Can you work these out from the model? Positions are in its coordinate system, mm. Face numbers are marked on the shaded views. A direction names the side the tool comes from. Coordinates: 2 decimals unless noted, no trailing zeros. Order: outer loops, then holes, each group sorted by start corner. A loop starts at its lowest first (then second) coordinate and runs counter-clockwise, first axis right, second up. Notation, with made-up numbers: (31, 0.25) -> (55, 0.25) arc R22 cw to (55, 18.25) -> close; hole circle Ø6 at (25, -16.5). An arc over 180 degrees is marked (long way). Answer in a Markdown table with one row per item. Add a question column.
1. We'd pull the mould along Z, two halves only. Please class the marked faces 1, 2, 3 and 4: pulls with the +Z half, pulls with the -Z half, needs draft (parallel to the pull), parting line crosses it, or undercut.
2. Imagine slicing it at C-C on z = 36. Write out the boundary of the cut face in (x, y).
3. Imagine slicing it at B-B on y = 45. Write out the boundary of the cut face in (x, z).
4. Imagine slicing it at A-A on x = 16. State how many separate pieces and enclosed holes the cut face has, plus the area to 4 significant figures.
5. Will these pins go through, and if not, where does the flat tip stop? pin 1 (10 mm diameter, centred on y = 33, z = 23.5, fed in from -X); pin 2 (3 mm diameter, centred on x = 22.5, z = 13.5, fed in from +Y); pin 3 (5 mm diameter, centred on x = 36, z = 16, fed in from -Y); pin 4 (2.5 mm diameter, centred on x = 16, y = 47.5, fed in from +Z).
6. Imagine slicing it at D-D on y = 27. Write out the boundary of the cut face in (x, z).
7. On a 3-axis mill with a long thin cutter (end or side, diameter ignored), from which of +Z, -Z, +X, -X, +Y, -Y can I reach the whole of each face in a straight line? I mean the marked faces 5 and 6. Say none if no direction works.
8. If I drill on line 1 along Z through (x, y) = (6.55, 16); line 2 along Z through (x, y) = (6.5, 29.5), over which ranges is the centre line in solid material (lowest first)? Write a range as [from, to].
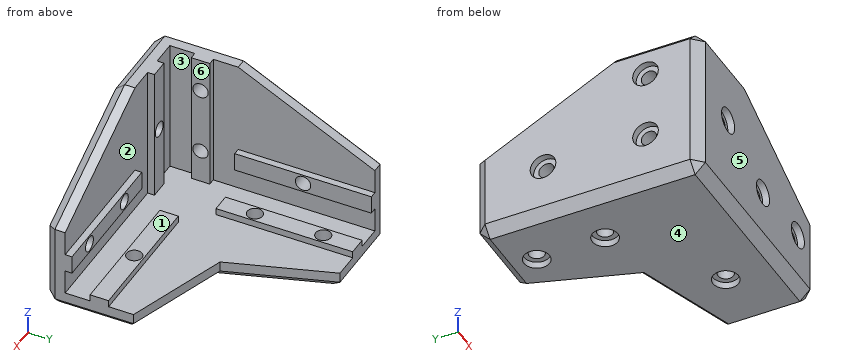
from build123d import *

# Parameters (mm, degrees)
F1_DEPTH  = 6
F3_DEPTH  = 20
F5_DEPTH  = 20
F7_DEPTH  = 40
F9_DEPTH  = 2
F11_DEPTH = 2
F13_DEPTH = 2
F14_R     = 2.25
F15_DEPTH = 8
F16_R     = 2.25
F17_DEPTH = 8
F18_R     = 2.25
F19_DEPTH = 8
F20_R     = 3.75
F21_DEPTH = 2
F22_R     = 3.75
F23_DEPTH = 2
F24_R     = 3.75
F25_DEPTH = 2
F27_DEPTH = 6
F29_DEPTH = 6
F31_DEPTH = 6
F32_SIZE  = 3


with BuildPart() as f1:
    # F0 (on Top) → F1 (new body)
    with BuildSketch(Plane.XY):
        Polygon((0, 66), (0, 0), (66, 0), (66, 26), (26, 26), (26, 66), align=None)
    extrude(amount=F1_DEPTH)

    # F2 (on face) → F3 (join)
    with BuildSketch(Plane.XY.offset(6)):
        Polygon((6, 66), (0, 66), (0, 0), (66, 0), (66, 6), (6, 6), align=None)
    extrude(amount=F3_DEPTH)

    # F4 (on face) → F5 (join)
    with BuildSketch(Plane.XY.offset(26)):
        Polygon((6, 6), (6, 26), (0, 26), (0, 0), (26, 0), (26, 6), align=None)
    extrude(amount=F5_DEPTH)

    # F6 (on face) → F7 (join)
    with BuildSketch(Plane.XY.offset(6)):
        Polygon((13.29, 6), (16, 6), (18.71, 6), (18.71, 8), (13.29, 8), align=None)
        Polygon((6, 18.71), (6, 16), (6, 13.29), (8, 13.29), (8, 18.71), align=None)
    extrude(amount=F7_DEPTH)

    # F8 (on face) → F9 (join)
    with BuildSketch(Plane.XY.offset(6)):
        Polygon((66, 13.29), (66, 16), (66, 18.71), (26, 18.71), (26, 13.29), align=None)
        Polygon((18.71, 66), (16, 66), (13.29, 66), (13.29, 26), (18.71, 26), align=None)
    extrude(amount=F9_DEPTH)

    # F10 (on face) → F11 (join)
    with BuildSketch(Plane(origin=(0, 6, 0), x_dir=(-1, 0, 0), z_dir=(0, 1, 0))):
        Polygon((-66, 18.71), (-66, 16), (-66, 13.29), (-26, 13.29), (-26, 16), (-26, 18.71), align=None)
    extrude(amount=F11_DEPTH)

    # F12 (on face) → F13 (join)
    with BuildSketch(Plane.YZ.offset(6)):
        Polygon((66, 13.29), (66, 16), (66, 18.71), (26, 18.71), (26, 13.29), align=None)
    extrude(amount=F13_DEPTH)

    # F14 (on face) → F15 (cut, through all)
    with BuildSketch(Plane.XZ):
        with Locations((56, 16)):
            Circle(F14_R)
        with Locations((16, 26)):
            Circle(F14_R)
        with Locations((36, 16)):
            Circle(F14_R)
    extrude(amount=-F15_DEPTH, mode=Mode.SUBTRACT)

    # F16 (on face) → F17 (cut, through all)
    with BuildSketch(Plane(origin=(0, 0, 0), x_dir=(0, -1, 0), z_dir=(-1, 0, 0))):
        with Locations((-16, 36)):
            Circle(F16_R)
        with Locations((-46, 16)):
            Circle(F16_R)
        with Locations((-16, 16)):
            Circle(F16_R)
    extrude(amount=-F17_DEPTH, mode=Mode.SUBTRACT)

    # F18 (on face) → F19 (cut, through all)
    with BuildSketch(Plane(origin=(0, 0, 0), x_dir=(1, 0, 0), z_dir=(0, 0, -1))):
        with Locations((46, -16)):
            Circle(F18_R)
        with Locations((16, -56)):
            Circle(F18_R)
        with Locations((16, -36)):
            Circle(F18_R)
    extrude(amount=-F19_DEPTH, mode=Mode.SUBTRACT)

    # F20 (on face) → F21 (cut)
    with BuildSketch(Plane.XZ):
        with Locations((16, 26)):
            Circle(F20_R)
        with Locations((36, 16)):
            Circle(F20_R)
        with Locations((56, 16)):
            Circle(F20_R)
    extrude(amount=-F21_DEPTH, mode=Mode.SUBTRACT)

    # F22 (on face) → F23 (cut)
    with BuildSketch(Plane(origin=(0, 0, 0), x_dir=(0, -1, 0), z_dir=(-1, 0, 0))):
        with Locations((-16, 36)):
            Circle(F22_R)
        with Locations((-46, 16)):
            Circle(F22_R)
        with Locations((-16, 16)):
            Circle(F22_R)
    extrude(amount=-F23_DEPTH, mode=Mode.SUBTRACT)

    # F24 (on face) → F25 (cut)
    with BuildSketch(Plane(origin=(0, 0, 0), x_dir=(1, 0, 0), z_dir=(0, 0, -1))):
        with Locations((16, -56)):
            Circle(F24_R)
        with Locations((46, -16)):
            Circle(F24_R)
        with Locations((16, -36)):
            Circle(F24_R)
    extrude(amount=-F25_DEPTH, mode=Mode.SUBTRACT)

    # F26 (on face) → F27 (join)
    with BuildSketch(Plane.XZ):
        Polygon((66, 26), (26, 46), (26, 26), align=None)
    extrude(amount=-F27_DEPTH)

    # F28 (on face) → F29 (join)
    with BuildSketch(Plane(origin=(0, 0, 0), x_dir=(0, -1, 0), z_dir=(-1, 0, 0))):
        Polygon((-26, 46), (-66, 26), (-26, 26), align=None)
    extrude(amount=-F29_DEPTH)

    # F30 (on face) → F31 (join)
    with BuildSketch(Plane(origin=(0, 0, 0), x_dir=(1, 0, 0), z_dir=(0, 0, -1))):
        Polygon((26, -26), (26, -66), (36, -36), (66, -26), align=None)
    extrude(amount=-F31_DEPTH)

    # F32
    f32_edges = [f1.edges().sort_by_distance(p)[0] for p in [
        (46, 0, 36),
        (13, 0, 46),
        (0, 13, 46),
        (0, 46, 36),
        (31, 51, 0),
        (51, 31, 0),
        (13, 66, 0),
        (66, 13, 0),
        (66, 0, 13),
        (0, 66, 13),
        (33, 0, 0),
        (0, 33, 0),
        (0, 0, 23),
    ]]
    chamfer(f32_edges, length=F32_SIZE)


solid = f1.part
Answers follow:
| question | item | result |
|---|---|---|
| 1 | face 1 | pulls with the +Z half |
| 1 | face 2 | undercut |
| 1 | face 3 | needs draft |
| 1 | face 4 | pulls with the -Z half |
| 2 | outline | (0, 3) -> (3, 0) -> (39.29, 0) -> (46, 3) -> (46, 6) -> (18.71, 6) -> (18.71, 8) -> (13.29, 8) -> (13.29, 6) -> (6, 6) -> (6, 13.29) -> (8, 13.29) -> (8, 13.75) -> (2, 13.75) -> (2, 12.25) -> (0, 12.25) -> close; (0, 19.75) -> (2, 19.75) -> (2, 18.25) -> (8, 18.25) -> (8, 18.71) -> (6, 18.71) -> (6, 46) -> (3, 46) -> (0, 39.29) -> close |
| 3 | outline | (0, 3) -> (3, 0) -> (29.84, 0) -> (33, 3) -> (33, 6) -> (18.71, 6) -> (18.71, 8) -> (13.29, 8) -> (13.29, 6) -> (6, 6) -> (6, 13.29) -> (8, 13.29) -> (8, 13.98) -> (2, 13.98) -> (2, 12.39) -> (0, 12.39) -> close; (0, 19.61) -> (2, 19.61) -> (2, 18.02) -> (8, 18.02) -> (8, 18.71) -> (6, 18.71) -> (6, 36.5) -> (3, 36.5) -> (0, 33.15) -> close |
| 4 | separate pieces | 4 |
| 4 | enclosed holes | 0 |
| 4 | area | 656.5 mm² |
| 5 | pin 1 | stops at x = 0 |
| 5 | pin 2 | stops at y = 6 |
| 5 | pin 3 | stops at y = 2 |
| 5 | pin 4 | stops at z = 8 |
| 6 | outline | (0, 3) -> (3, 0) -> (53.51, 0) -> (63, 3) -> (63, 6) -> (18.71, 6) -> (18.71, 8) -> (13.29, 8) -> (13.29, 6) -> (6, 6) -> (6, 13.29) -> (8, 13.29) -> (8, 18.71) -> (6, 18.71) -> (6, 45.5) -> (3, 45.5) -> (0, 42.15) -> close |
| 7 | face 5 | +Z, -Z, +X, -X, -Y |
| 7 | face 6 | +Z, +Y |
| 8 | line 1 | z = [0, 13.75], [18.25, 33.75], [38.25, 46] |
| 8 | line 2 | z = [0, 6], [13.29, 18.71] |
